Geometry check sheet. Reference: the model listing, model coordinates, mm. Round coordinates to 2 decimals unless told otherwise and drop trailing zeros. Order: outer loops, then holes, each group sorted by start corner. A loop starts at its lowest first (then second) coordinate and runs counter-clockwise, first axis right, second up. Notation, with made-up numbers: (52, 0.5) - (98, 0.5) arc R37 ccw to (98, 38.5) - close; hole circle Ø11 at (70, 8.25). An arc over 180 degrees is marked (long way). Return JSON: item names as keys, results as strings. Group by question number.
Q1. Material ranges on line 1 along Y through (x, z) = (405, 4.75); line 2 along X through (y, z) = (45.5, 12.25); line 3 along Y through (x, z) = (295, 15.5), recorded low to high.
Q2. Sectioned sample at B-B, the plane x = 185. Record the cut outline in (y, z).
Q3. Sectioned sample at A-A, the plane y = 85. Record the cut outline in (x, z).
Q4. Sectioned sample at C-C, the plane z = 9.25. Record the cut outline in (x, y), then the cut area to 3 significant figures.
```python
from build123d import *

# Parameters (mm, degrees)
F0_W     = 450
F0_H     = 120
F1_DEPTH = 20
F3_D     = 24
F4_SIZE  = 5


with BuildPart() as f1:
    # F0 (on Top) → F1 (new body)
    with BuildSketch(Plane.XY):
        with Locations((225, 60)):
            Rectangle(F0_W, F0_H)
    extrude(amount=F1_DEPTH)

    # F3 (through all)
    with Locations(Plane.XY.offset(20)):
        with Locations((185, 85), (185, 35), (295, 85), (295, 35), (405, 85), (405, 35)):
            Hole(F3_D / 2)

    # F4
    f4_edges = [f1.edges().sort_by_distance(p)[0] for p in [
        (225, 120, 20),
        (225, 0, 20),
        (0, 60, 20),
    ]]
    chamfer(f4_edges, length=F4_SIZE)


solid = f1.part
```
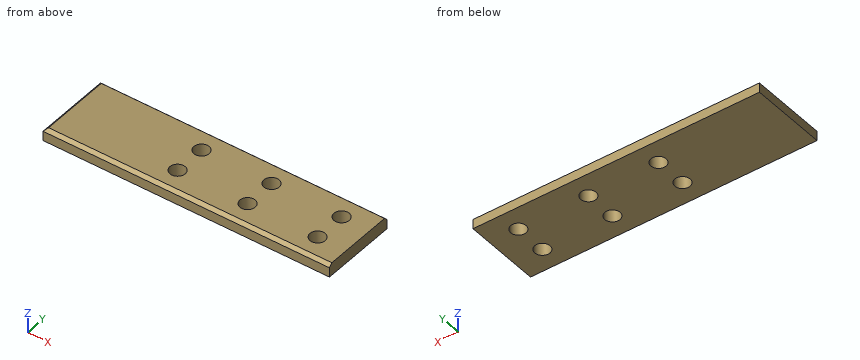
Reply:
{
 "1": {"line 1": "0 to 23, 47 to 73, 97 to 120", "line 2": "0 to 179.19, 190.81 to 289.19, 300.81 to 399.19, 410.81 to 450", "line 3": "0.5 to 23, 47 to 73, 97 to 119.5"},
 "2": {"outline": "(0, 0) - (23, 0) - (23, 20) - (5, 20) - (0, 15) - close; (47, 0) - (73, 0) - (73, 20) - (47, 20) - close; (97, 0) - (120, 0) - (120, 15) - (115, 20) - (97, 20) - close"},
 "3": {"outline": "(0, 0) - (173, 0) - (173, 20) - (5, 20) - (0, 15) - close; (197, 0) - (283, 0) - (283, 20) - (197, 20) - close; (307, 0) - (393, 0) - (393, 20) - (307, 20) - close; (417, 0) - (450, 0) - (450, 20) - (417, 20) - close"},
 "4": {"outline": "(0, 0) - (450, 0) - (450, 120) - (0, 120) - close; hole circle Ø24 at (185, 35); hole circle Ø24 at (185, 85); hole circle Ø24 at (295, 35); hole circle Ø24 at (295, 85); hole circle Ø24 at (405, 35); hole circle Ø24 at (405, 85)", "area": "51,300 mm^2"}
}
